Answer from the drawing. Dimensions are ordinates in mm from the lowest x, y and z of the part. A direction names the side the tool comes from. Round coordinates to 2 decimals unless told otherwise and drop trailing zeros. Write each loop counter-clockwise with the first axis right and the second up, starting at its lowest first coordinate (ties: lowest second). Pieces come first, ordered by that corner, then holes. Notation, with made-up numbers: M 85,73.25 L 90,73.25 A28 cw 90,94.25 Z; hole C 72.25,-39.75 d4. An arc over 180 degrees is marked long. Answer as CSV lines item,"result". Start each with the question number.
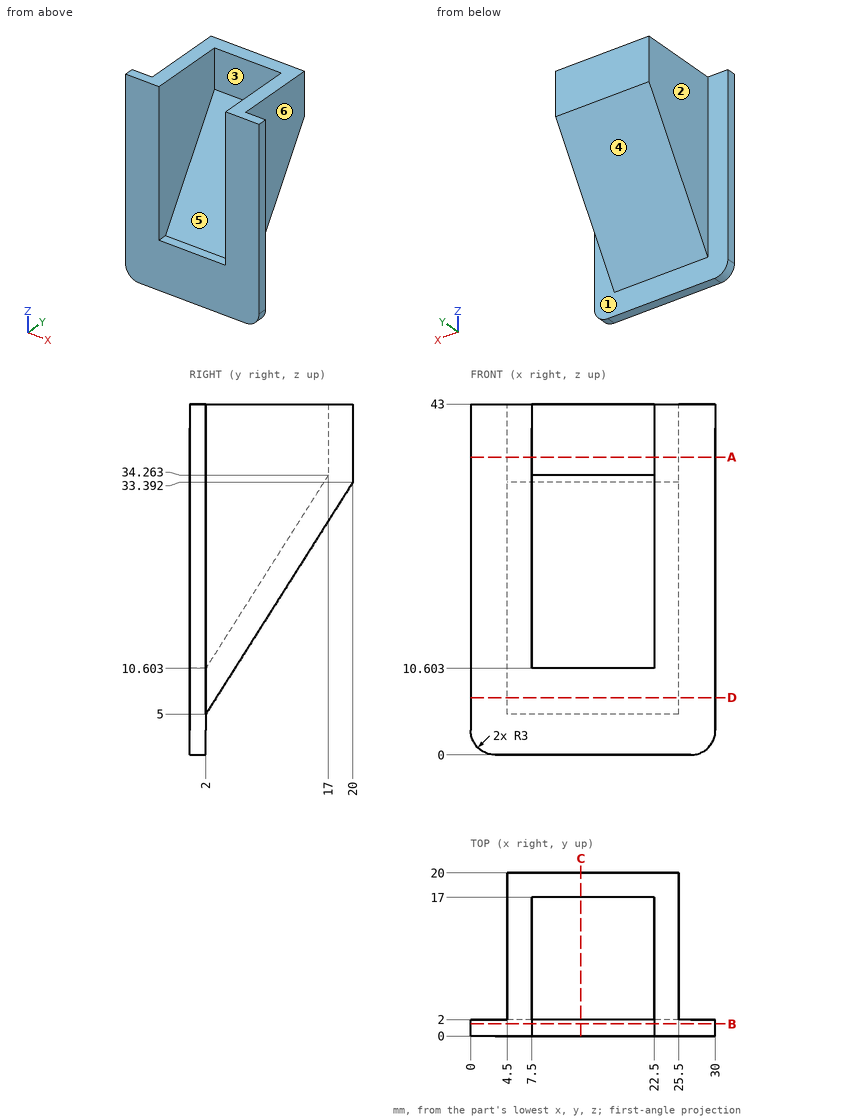
Q1. Find section C-C (x = 13.5). Determine the outline of the cut face in (y, z), plus the area to 3 significant figures.
Q2. Find section B-B (y = 1.5). Determine the outline of the cut face in (x, z).
Q3. Find section D-D (z = 7). Determine the outline of the cut face in (x, y).
Q4. For the marked faces 1, 2 and 3, determine the directions among +Z, -Z, +X, -X, +Y, -Y from which every point of the face is accessible in a straight line to the end or side of a thin tool.
Q5. Straight lines are drawn through the part: L1, parallel to X at y = 4.5, z = 19; L2, parallel to X at y = 1.5, z = 24; L3, parallel to X at y = 18.75, z = 37. For each, find the intervals that lie inside material, in ascending order.
Q6. Each of these flat-tipped pins is pushed along its axis until it touches: P1, Ø7, axis at x = 12, z = 38.5, coming from the -Y side; P2, Ø4, axis at x = 26.5, y = 12, coming from the +Z side; P3, Ø5.5, axis at y = 11, z = 23.5, coming from the +X side; P4, Ø2, axis at x = 21.5, z = 18, coming from the +Y side (1 decimal). Where does it stop, or does it pass through?
Q7. The mould has two halves that part along X. Classify the marked faces 4, 5 and 6: +X half, -X half, draft (parallel to the pull), parting line (faces both ways), or undercut.
Q8. Find section A-A (z = 36.5). Determine the outline of the cut face in (x, y), plus the area to 3 significant figures.
Reported:
1,outline,"M 0,0 L 2,0 L 2,5 L 20,33.39 L 20,43 L 17,43 L 17,34.26 L 2,10.6 L 0,10.6 Z"
1,area,"141 mm2"
2,outline,"M 0,3 A3 ccw 3,0 L 27,0 A3 ccw 30,3 L 30,43 L 22.5,43 L 22.5,10.6 L 7.5,10.6 L 7.5,43 L 0,43 Z"
3,outline,"M 0,0 L 30,0 L 30,2 L 25.5,2 L 25.5,3.27 L 4.5,3.27 L 4.5,2 L 0,2 Z"
4,face 1,"-Z, +Y"
4,face 2,"+Z, -Z, -X, +Y"
4,face 3,"+Z, -Y"
5,L1,"x = 4.5 to 7.5, 22.5 to 25.5"
5,L2,"x = 0 to 7.5, 22.5 to 30"
5,L3,"x = 4.5 to 25.5"
6,P1,"stops at y = 17"
6,P2,"stops at z = 43"
6,P3,"stops at x = 25.5"
6,P4,"stops at y = 10.9"
7,face 4,"draft"
7,face 5,"undercut"
7,face 6,"+X half"
8,outline,"M 0,0 L 7.5,0 L 7.5,17 L 22.5,17 L 22.5,0 L 30,0 L 30,2 L 25.5,2 L 25.5,20 L 4.5,20 L 4.5,2 L 0,2 Z"
8,area,"183 mm2"
